```python
from build123d import *

# Parameters (mm, degrees)
SZKIC1_W                    = 115
SZKIC1_H                    = 115
DODANIE_WYCI_GNI_CIE1_DEPTH = 3
DODANIE_WYCI_GNI_CIE2_DEPTH = 6
SZKIC5_R                    = 2.1
WYTNIJ_WYCI_GNI_CIE1_DEPTH  = 163.833695476
SZKIC6_R                    = 1
WYTNIJ_WYCI_GNI_CIE2_DEPTH  = 10
ZAOKR_GLENIE1_R             = 20
SZKIC7_W                    = 15
SZKIC7_H                    = 10
WYTNIJ_WYCI_GNI_CIE3_DEPTH  = 1
WYTNIJ_WYCI_GNI_CIE4_DEPTH  = 10
SZKIC9_R                    = 1.1
WYTNIJ_WYCI_GNI_CIE5_DEPTH  = 132.613306252
SZKIC10_R                   = 1.1
WYTNIJ_WYCI_GNI_CIE6_DEPTH  = 10
DODANIE_WYCI_GNI_CIE4_DEPTH = 8
SZKIC14_W                   = 6
SZKIC14_H                   = 6
WYTNIJ_WYCI_GNI_CIE8_DEPTH  = 8
ZAOKR_GLENIE3_R             = 4
DODANIE_WYCI_GNI_CIE5_DEPTH = 8
SZKIC16_W                   = 6
SZKIC16_H                   = 6
WYTNIJ_WYCI_GNI_CIE9_DEPTH  = 8
ZAOKR_GLENIE5_R             = 4
SZYK_START                  = 27.034271247
SZYK_LINIOWY1_DEPTH         = 2.5


# Read off the part's stored shape, not the designer's step: Szyk liniowy1
with BuildPart() as part:
    # Szkic1 → Dodanie-wyciągnięcie1 (new body)
    with BuildSketch(Plane.XY):
        with Locations((57.5, -57.5)):
            Rectangle(SZKIC1_W, SZKIC1_H)
    extrude(amount=DODANIE_WYCI_GNI_CIE1_DEPTH)

    # Szkic3 → Dodanie-wyciągnięcie2 (add)
    with BuildSketch(Plane(origin=(115, 0, 0), x_dir=(0, 0, -1), z_dir=(1, 0, 0))):
        with BuildLine():
            Line((0, -51.5), (3.050613798, -51.5))
            ThreePointArc((3.050613798, -51.5), (8.050613798, -56.5), (3.050613798, -61.5))
            Line((3.050613798, -61.5), (0, -61.5))
            Line((0, -61.5), (0, -51.5))
        make_face()
    dodanie_wyci_gni_cie2 = extrude(amount=-DODANIE_WYCI_GNI_CIE2_DEPTH)

    # Lustro1: Dodanie-wyciągnięcie2 across plane
    add(dodanie_wyci_gni_cie2.mirror(Plane(origin=(57.5, 0, 0), x_dir=(0, 0, 1), z_dir=(1, 0, 0))))

    # Szkic5 → Wytnij-wyciągnięcie1 (cut, through all)
    with BuildSketch(Plane(origin=(115, 0, 0), x_dir=(0, 0, -1), z_dir=(1, 0, 0))):
        with Locations(Location((3.050613798, -56.5, 0), (0, 0, 90))):
            Circle(SZKIC5_R)
    extrude(amount=-WYTNIJ_WYCI_GNI_CIE1_DEPTH, mode=Mode.SUBTRACT)

    # Szkic6 → Wytnij-wyciągnięcie2 (cut)
    with BuildSketch(Plane.XY.offset(3)):
        with Locations((54.5, -112.5)):
            Circle(SZKIC6_R)
        with Locations((60.5, -112.5)):
            Circle(SZKIC6_R)
    extrude(amount=-WYTNIJ_WYCI_GNI_CIE2_DEPTH, mode=Mode.SUBTRACT)

    # Zaokrąglenie1
    zaokr_glenie1_edges = [part.edges().sort_by_distance(p)[0] for p in [
        (0, 0, 1.5),
        (115, 0, 1.5),
        (115, -115, 1.5),
        (0, -115, 1.5),
    ]]
    fillet(zaokr_glenie1_edges, radius=ZAOKR_GLENIE1_R)

    # Szkic7 → Wytnij-wyciągnięcie3 (cut)
    with BuildSketch(Plane.XY.offset(3)):
        with Locations((57.5, -110)):
            Rectangle(SZKIC7_W, SZKIC7_H)
    extrude(amount=-WYTNIJ_WYCI_GNI_CIE3_DEPTH, mode=Mode.SUBTRACT)

    # Szkic8 → Wytnij-wyciągnięcie4 (cut)
    with BuildSketch(Plane(origin=(0, 0, 0), x_dir=(-1, 0, 0), z_dir=(0, 0, -1))):
        with BuildLine():
            Line((-87.5, -97.5), (-27.5, -97.5))
            ThreePointArc((-27.5, -97.5), (-20.428932188, -94.571067812), (-17.5, -87.5))
            Line((-17.5, -87.5), (-17.5, -27.5))
            ThreePointArc((-17.5, -27.5), (-20.428932188, -20.428932188), (-27.5, -17.5))
            Line((-27.5, -17.5), (-87.5, -17.5))
            ThreePointArc((-87.5, -17.5), (-94.571067812, -20.428932188), (-97.5, -27.5))
            Line((-97.5, -27.5), (-97.5, -87.5))
            ThreePointArc((-97.5, -87.5), (-94.571067812, -94.571067812), (-87.5, -97.5))
        make_face()
    extrude(amount=-WYTNIJ_WYCI_GNI_CIE4_DEPTH, mode=Mode.SUBTRACT)

    # Szkic9 → Wytnij-wyciągnięcie5 (cut, through all)
    with BuildSketch(Plane(origin=(0, -51.5, 0), x_dir=(1, 0, 0), z_dir=(0, 1, 0))):
        with Locations(Location((3, 3.050613798, 0), (0, 0, 180))):
            Circle(SZKIC9_R)
    extrude(amount=-WYTNIJ_WYCI_GNI_CIE5_DEPTH, mode=Mode.SUBTRACT)

    # Szkic10 → Wytnij-wyciągnięcie6 (cut)
    with BuildSketch(Plane(origin=(0, -51.5, 0), x_dir=(1, 0, 0), z_dir=(0, 1, 0))):
        with Locations(Location((112, 3.050613798, 0), (0, 0, 180))):
            Circle(SZKIC10_R)
    extrude(amount=-WYTNIJ_WYCI_GNI_CIE6_DEPTH, mode=Mode.SUBTRACT)

    # Szkic13 → Dodanie-wyciągnięcie4 (add)
    with BuildSketch(Plane(origin=(0, 2.663945597, 0), x_dir=(-1, 0, 0), z_dir=(0, 0, -1))):
        Polygon((-53.080582618, -103.598349571), (-60.151650429, -110.669417382), (-61.919417382, -108.901650429), (-54.848349571, -101.830582618), align=None)
    extrude(amount=DODANIE_WYCI_GNI_CIE4_DEPTH)

    # Szkic14 → Wytnij-wyciągnięcie8 (cut)
    with BuildSketch(Plane(origin=(-25.258883476, -22.594937879, 0), x_dir=(-0.7071067811865481, 0.707106781186547, 0), z_dir=(-0.707106781186547, -0.7071067811865481, 0))):
        with Locations((-115.788735419, 3)):
            Rectangle(SZKIC14_W, SZKIC14_H)
    extrude(amount=-WYTNIJ_WYCI_GNI_CIE8_DEPTH, mode=Mode.SUBTRACT)

    # Zaokrąglenie3
    # the kernel refuses this fillet: 4 mm, written as the material it adds along each edge
    with BuildSketch(Plane(origin=(58.737436867, -106.591258223, -6), x_dir=(0, 0, 1), z_dir=(0.707106781186547, 0.7071067811865481, 0)), Plane(origin=(54.49479618, -102.348617536, -6), x_dir=(0.7071067811865481, -0.707106781186547, 0), z_dir=(0.707106781186547, 0.7071067811865481, 0))) as zaokr_glenie3_piece_1:
        with BuildLine():
            CenterArc((ZAOKR_GLENIE3_R, -ZAOKR_GLENIE3_R), ZAOKR_GLENIE3_R, 90, 90)
            Line((0, -ZAOKR_GLENIE3_R), (0, 0))
            Line((0, 0), (ZAOKR_GLENIE3_R, 0))
        make_face()
    extrude(amount=2.5)
    # the kernel refuses this fillet: 4 mm, written as the material it takes off along each edge
    with BuildSketch(Plane(origin=(53.080582618, -115.076539597, -8), x_dir=(0, 0, 1), z_dir=(0.7071067811865476, 0.7071067811865476, 0)), Plane(origin=(61.919417382, -92.095569208, -8), x_dir=(0, 0, 1), z_dir=(-0.7071067811865476, -0.7071067811865476, 0))) as zaokr_glenie3_2_piece_1:
        with BuildLine():
            CenterArc((ZAOKR_GLENIE3_R, -ZAOKR_GLENIE3_R), ZAOKR_GLENIE3_R, 90, 90)
            Line((0, -ZAOKR_GLENIE3_R), (0, 0))
            Line((0, 0), (ZAOKR_GLENIE3_R, 0))
        make_face()
    extrude(amount=22.5, mode=Mode.SUBTRACT)

    # Szkic15 → Dodanie-wyciągnięcie5 (add)
    with BuildSketch(Plane(origin=(0, 0, 0), x_dir=(-1, 0, 0), z_dir=(0, 0, -1))):
        Polygon((-104.697591975, -106.465358928), (-106.465358928, -104.697591975), (-99.394291117, -97.626524164), (-97.626524164, -99.394291117), align=None)
    extrude(amount=DODANIE_WYCI_GNI_CIE5_DEPTH)

    # Szkic16 → Wytnij-wyciągnięcie9 (cut)
    with BuildSketch(Plane(origin=(-0.883883476, -0.883883476, 0), x_dir=(-0.7071067811865475, 0.7071067811865477, 0), z_dir=(-0.7071067811865477, -0.7071067811865475, 0))):
        with Locations((-144.31475452, 3)):
            Rectangle(SZKIC16_W, SZKIC16_H)
    extrude(amount=-WYTNIJ_WYCI_GNI_CIE9_DEPTH, mode=Mode.SUBTRACT)

    # Zaokrąglenie5
    # the kernel refuses this fillet: 4 mm, written as the material it adds along each edge
    with BuildSketch(Plane(origin=(99.040737726, -100.808504679, -6), x_dir=(0.7071067811865475, -0.7071067811865477, 0), z_dir=(0.7071067811865477, 0.7071067811865475, 0)), Plane(origin=(103.283378413, -105.051145366, -6), x_dir=(0, 0, 1), z_dir=(0.7071067811865477, 0.7071067811865475, 0))) as zaokr_glenie5_piece_1:
        with BuildLine():
            CenterArc((ZAOKR_GLENIE5_R, -ZAOKR_GLENIE5_R), ZAOKR_GLENIE5_R, 90, 90)
            Line((0, -ZAOKR_GLENIE5_R), (0, 0))
            Line((0, 0), (ZAOKR_GLENIE5_R, 0))
        make_face()
    extrude(amount=2.5)
    # the kernel refuses this fillet: 4 mm, written as the material it takes off along each edge
    with BuildSketch(Plane(origin=(106.465358928, -90.555456352, -8), x_dir=(0, 0, 1), z_dir=(-0.7071067811865476, -0.7071067811865476, 0)), Plane(origin=(97.626524164, -113.53642674, -8), x_dir=(0, 0, 1), z_dir=(0.7071067811865476, 0.7071067811865476, 0))) as zaokr_glenie5_2_piece_1:
        with BuildLine():
            CenterArc((ZAOKR_GLENIE5_R, -ZAOKR_GLENIE5_R), ZAOKR_GLENIE5_R, 90, 90)
            Line((0, -ZAOKR_GLENIE5_R), (0, 0))
            Line((0, 0), (ZAOKR_GLENIE5_R, 0))
        make_face()
    extrude(amount=22.5, mode=Mode.SUBTRACT)

    # Szyk liniowy1 outline → Szyk liniowy1 (add)
    with BuildSketch(Plane(origin=(0, 0, 0), x_dir=(0.7071067811865471, -0.707106781186548, 0), z_dir=(0.707106781186548, 0.707106781186547, 0)).offset(SZYK_START)):
        with BuildLine():
            ThreePointArc((121.030483272, 4), (119.858910397, 6.828427125), (117.030483272, 8))
            Line((117.030483272, 8), (115.030483272, 8))
            ThreePointArc((115.030483272, 8), (112.202056147, 6.828427125), (111.030483272, 4))
            Line((111.030483272, 4), (111.030483272, 0))
            Line((111.030483272, 0), (113.030483272, 0))
            Line((113.030483272, 0), (113.030483272, 2))
            ThreePointArc((113.030483272, 2), (113.868205612, 4.449489743), (116.030483272, 5.872983346))
            ThreePointArc((116.030483272, 5.872983346), (118.192760932, 4.449489743), (119.030483272, 2))
            Line((119.030483272, 2), (119.030483272, 0))
            Line((119.030483272, 0), (121.030483272, 0))
            Line((121.030483272, 0), (121.030483272, 4))
        make_face()
    extrude(amount=SZYK_LINIOWY1_DEPTH)


solid = part.part
```
Here's how the part is built. I have some questions about the finished solid (model axes, mm). A direction names the side the tool comes from. Give positions to 0.01 mm unless a question says otherwise; leave off trailing zeros. Order: outer loops, then holes, each group sorted by start corner. A loop starts at its lowest first (then second) coordinate and runs counter-clockwise, first axis right, second up. Notation, with made-up numbers: M -26,44.25 L -21,44.25 A6 cw -21,49.25 Z; hole C 24,67 d8. An arc over 180 degrees is marked long. Use a Markdown table: item, result. Add a question column.
1. If we mould it in two halves opening along Y, with no side actions, what happens to faces 5 (the flat face through (102, -62, -8)), 6 (the flat face through (57.451, -105.305, -5.722)), 7 (the flat face through (97.5, -57, 1)), 8 (the cylindrical face through (94.65, -94.49, 1.48))? For each: +Y half, -Y half, draft (parallel to the pull), parting line (faces both ways), or undercut.
2. Suppose I cut it at B-B (y = -93). List the corners of the cut face in (x, z) for me.
3. For pin 1 Ø3 at (x, z) = (3, -3.05) entering from -Y; pin 2 Ø0.5 at (x, z) = (56.5, 2.5) entering from -Y; pin 3 Ø2.5 at (x, y) = (54.5, -112.5) entering from +Z, each with a flat end and sliding along its axis, tell me the tip position at first contact or that it passes through.
4. Suppose I cut it at A-A (x = 39). List the corners of the cut face in (y, z) for me, and give its area (3 significant figures).
5. On a 3-axis mill with a long thin cutter (end or side, diameter ignored), from which of +Z, -Z, +X, -X, +Y, -Y can I reach the whole of each face in a straight line? I mean faces 1 (the cylindrical face through (3.042, -58.048, -1.631)), 2 (the flat face through (57.65, -101.97, -5.72)), 3 (the cylindrical face through (20.35, -20.51, 1.48)), 4 (the flat face through (109, -58, -5)). Say none if no direction works.
6. I need wall thicknesses on probe 1 along Y at (x, z) = (60.5, 0.4); probe 2 along Y at (x, z) = (71, 2.5); probe 3 along X at (y, z) = (-112.5, 0.5). Which ranges of each line are inside material? Lowest first, please. Write a range as from..to.
Results list:
| question | item | result |
|---|---|---|
| 1 | face 5 | draft |
| 1 | face 6 | -Y half |
| 1 | face 7 | undercut |
| 1 | face 8 | undercut |
| 2 | outline | M 0,0 L 19.15,0 L 19.15,3 L 0,3 Z; M 95.85,0 L 115,0 L 115,3 L 95.85,3 Z |
| 3 | pin 1 | stops at y = -61.5 |
| 3 | pin 2 | stops at y = -105 |
| 3 | pin 3 | stops at z = 2 |
| 4 | outline | M -115,0 L -97.5,0 L -97.5,3 L -115,3 Z; M -17.5,0 L 0,0 L 0,3 L -17.5,3 Z |
| 4 | area | 105 mm² |
| 5 | face 1 | -X |
| 5 | face 2 | -Z, +Y |
| 5 | face 3 | +Z, -Z |
| 5 | face 4 | -Z, +Y, -Y |
| 6 | probe 1 | y = -115..-113.5, -111.5..-97.5, -17.5..0 |
| 6 | probe 2 | y = -115..-97.5, -17.5..0 |
| 6 | probe 3 | x = 10.32..53.5, 55.5..59.5, 61.5..104.68 |
